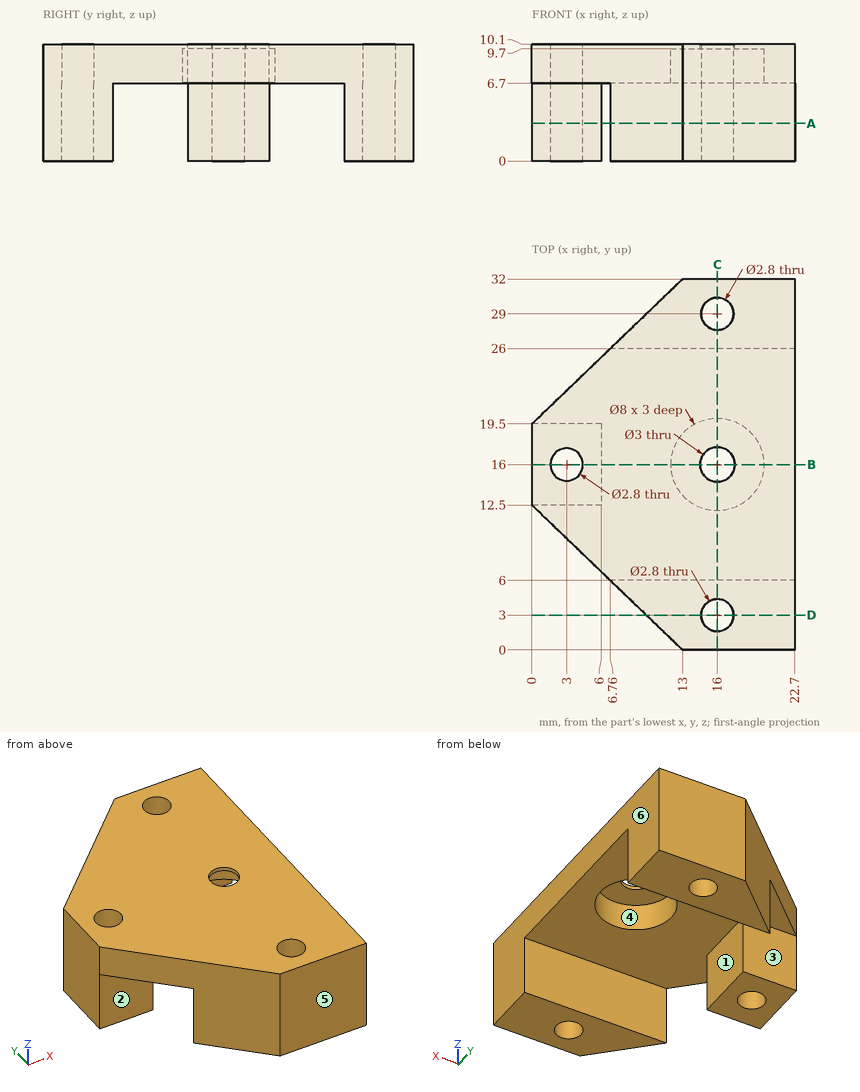
Here's the drawing with two shaded views (mm, measured from the low corner). I have some questions. A direction names the side the tool comes from. Round coordinates to 2 decimals unless told otherwise and drop trailing zeros. Order: outer loops, then holes, each group sorted by start corner. A loop starts at its lowest first (then second) coordinate and runs counter-clockwise, first axis right, second up. Notation, with made-up numbers: (7.5, 54.25) -> (30.5, 54.25) arc R20 cw to (30.5, 74.25) -> close; hole circle Ø7 at (80.5, 66). An arc over 180 degrees is marked (long way). Write each question's results on one line, items separated by ' | '. Start each with the question number.
Item 1: If we section it at B-B, the plane y = 16: Write out the boundary of the cut face in (x, z).
Item 2: Thinking about a two-plate mould opening in Y: for the marked faces 4, 5 and 6, which applies, +Y half, -Y half, draft (parallel to the pull), parting line (faces both ways), or undercut?
Item 3: If we section it at C-C, the plane x = 16: Write out the boundary of the cut face in (y, z), then the cut area to 3 significant figures.
Item 4: If we section it at D-D, the plane y = 3: Write out the boundary of the cut face in (x, z).
Item 5: Please list where these lines run through material, in increasing order: L1, parallel to Y at x = 16, z = 7; L2, parallel to Y at x = 19.75, z = 5.75; L3, parallel to Y at x = 16, z = 9.95.
Item 6: If we section it at A-A, the plane z = 3.25: Write out the boundary of the cut face in (x, y), then the cut area to 3 significant figures.
Item 7: Will these pins go through, and if not, where does the flat tip stop? pin 1 (1.8 mm diameter, centred on x = 2.5, z = 3.5, fed in from +Y); pin 2 (13 mm diameter, centred on x = 16, y = 16, fed in from -Z); pin 3 (3.5 mm diameter, centred on y = 15.5, z = 3, fed in from +X).
Item 8: Which directions (+Z, -Z, +X, -X, +Y, -Y) give clear straight access to the entire face, cutting with the end or side of a thin tool? Please do the marked faces 1, 2 and 3.
Results:
1) outline: (0, 0) -> (1.6, 0) -> (1.6, 10.1) -> (0, 10.1) -> close; (4.4, 0) -> (6, 0) -> (6, 6.7) -> (12, 6.7) -> (12, 9.7) -> (14.5, 9.7) -> (14.5, 10.1) -> (4.4, 10.1) -> close; (17.5, 9.7) -> (20, 9.7) -> (20, 6.7) -> (22.7, 6.7) -> (22.7, 10.1) -> (17.5, 10.1) -> close
2) face 4: undercut | face 5: -Y half | face 6: draft
3) outline: (0, 0) -> (1.6, 0) -> (1.6, 10.1) -> (0, 10.1) -> close; (4.4, 0) -> (6, 0) -> (6, 6.7) -> (12, 6.7) -> (12, 9.7) -> (14.5, 9.7) -> (14.5, 10.1) -> (4.4, 10.1) -> close; (17.5, 9.7) -> (20, 9.7) -> (20, 6.7) -> (26, 6.7) -> (26, 0) -> (27.6, 0) -> (27.6, 10.1) -> (17.5, 10.1) -> close; (30.4, 0) -> (32, 0) -> (32, 10.1) -> (30.4, 10.1) -> close | area: 107 mm2
4) outline: (9.88, 0) -> (14.6, 0) -> (14.6, 10.1) -> (9.88, 10.1) -> close; (17.4, 0) -> (22.7, 0) -> (22.7, 10.1) -> (17.4, 10.1) -> close
5) L1: y = 0 to 1.6, 4.4 to 12, 20 to 27.6, 30.4 to 32 | L2: y = 0 to 6, 26 to 32 | L3: y = 0 to 1.6, 4.4 to 14.5, 17.5 to 27.6, 30.4 to 32
6) outline: (0, 12.5) -> (6, 12.5) -> (6, 19.5) -> (0, 19.5) -> close; (6.76, 6) -> (13, 0) -> (22.7, 0) -> (22.7, 6) -> close; (6.76, 26) -> (22.7, 26) -> (22.7, 32) -> (13, 32) -> close; hole circle Ø2.8 at (3, 16); hole circle Ø2.8 at (16, 3); hole circle Ø2.8 at (16, 29) | area: 177 mm2
7) pin 1: stops at y = 19.5 | pin 2: stops at z = 6.7 | pin 3: stops at x = 6
8) face 1: -Z, +X, +Y, -Y | face 2: -Z, +X, -X, -Y | face 3: -Z, +X, -X, +Y
